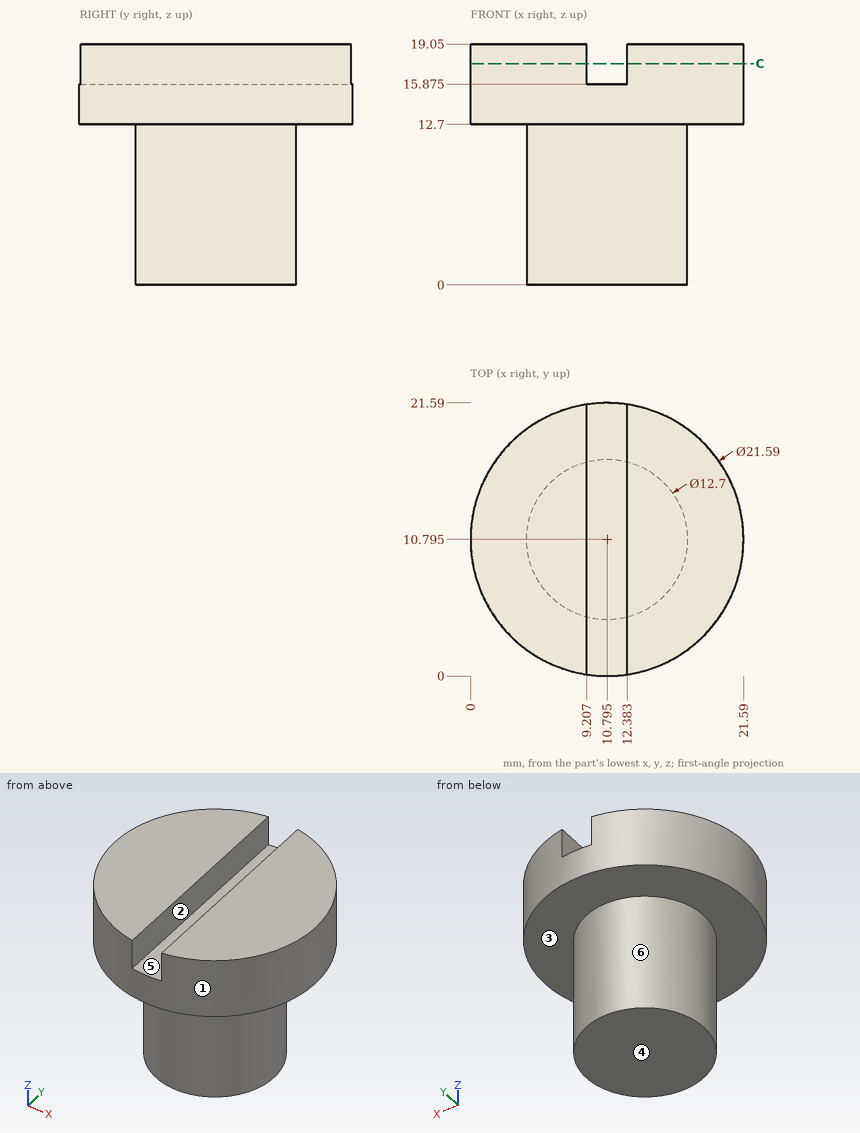
Source: three-view drawing plus pictorial views. Frame: mm from the lowest corner of the part. A direction names the side the tool comes from. Give positions to 0.01 mm unless a question says otherwise; leave off trailing zeros. Order: outer loops, then holes, each group sorted by start corner. A loop starts at its lowest first (then second) coordinate and runs counter-clockwise, first axis right, second up. Notation, with made-up numbers: (3.5, 47.5) -> (62.5, 47.5) arc R22 cw to (62.5, 72.5) -> close; hole circle Ø2 at (52.5, 84). An arc over 180 degrees is marked (long way). Write each question's results on one line, items separated by ' | '. Start each with the question number.
Item 1: Contact query for flat-ended pins moving along their axis: P1, Ø4, axis at y = 7.5, z = 10.5, coming from the -X side; P2, Ø3, axis at x = 18.5, y = 7.5, coming from the -Z side. Output: stop coordinate, or through.
Item 2: Mould query, pull axis X, two halves, no side actions, for the marked faces 1, 2 and 3. Classes: pulls with the +X half, pulls with the -X half, needs draft (parallel to the pull), parting line crosses it, or undercut.
Item 3: Line query: line 1 (Z direction, x = 16, y = 5.75); line 2 (Z direction, x = 12.25, y = 13.75) (1 decimal); line 3 (Y direction, x = 10.75, z = 8.5) (1 decimal). Output: solid intervals per line, ascending.
Item 4: Set-up query: the marked faces 4, 5 and 6. Return all of +Z, -Z, +X, -X, +Y, -Y with unobstructed straight access to the full face (end or side cutting, diameter ignored); none if empty.
Item 5: Cut plane C-C on z = 17.5. Return the cut outline in (x, y) (1 decimal), then the cut area to 3 significant figures.
Established:
1) P1: x = 4.58 | P2: z = 12.7
2) face 1: parting line crosses it | face 2: undercut | face 3: needs draft
3) line 1: 12.7 to 19.05 | line 2: 0 to 15.9 | line 3: 4.4 to 17.1
4) face 4: -Z, +X, -X, +Y, -Y | face 5: +Z, +Y, -Y | face 6: -Z
5) outline: (9.2, 0.1) -> (9.2, 21.5) arc R10.8 ccw to start; (12.4, 0.1) arc R10.8 ccw to (12.4, 21.5) -> close | area: 298 mm^2
